Can you work these out from the drawing? Everything is in mm from the part's minimum corner. Coordinates: 2 decimals unless noted, no trailing zeros. Order: outer loops, then holes, each group sorted by start corner. A loop starts at its lowest first (then second) coordinate and runs counter-clockwise, first axis right, second up. Notation, with made-up numbers: (29.5, 39) -> (54.5, 39) arc R30 cw to (54.5, 71) -> close; hole circle Ø7 at (71, 56.25). An arc over 180 degrees is marked (long way). Return JSON: item names as keys, results as strings. Group by question number.
1) If I drill on probe 1 along X at (y, z) = (5.75, 35.5) (1 decimal); probe 2 along X at (y, z) = (1.5, 33.5) (1 decimal); probe 3 along X at (y, z) = (10.5, 38) (1 decimal), over which ranges is the centre line in solid material (lowest first)? Write a range as from..to.
2) For pin 1 (3 mm diameter, centred on x = 49.5, y = 11.5, fed in from +Z) (1 decimal); pin 2 (5 mm diameter, centred on y = 2.5, z = 52.5, fed in from +X); pin 3 (1.5 mm diameter, centred on y = 6, z = 30.5, fed in from -X), each with a flat end and sliding along its axis, tell me the tip position at first contact or that it passes through.
3) If we section it at B-B, the plane y = 12.25: Please give me the cut outline in (x, z).
4) Thinking about a two-plate mould opening in X: for the marked faces 1, 2 and 3, which applies, +X half, -X half, draft (parallel to the pull), parting line (faces both ways), or undercut?
5) If we section it at A-A, the plane y = 1.25: Please give me the cut outline in (x, z) (1 decimal), then the cut area to 3 significant figures.
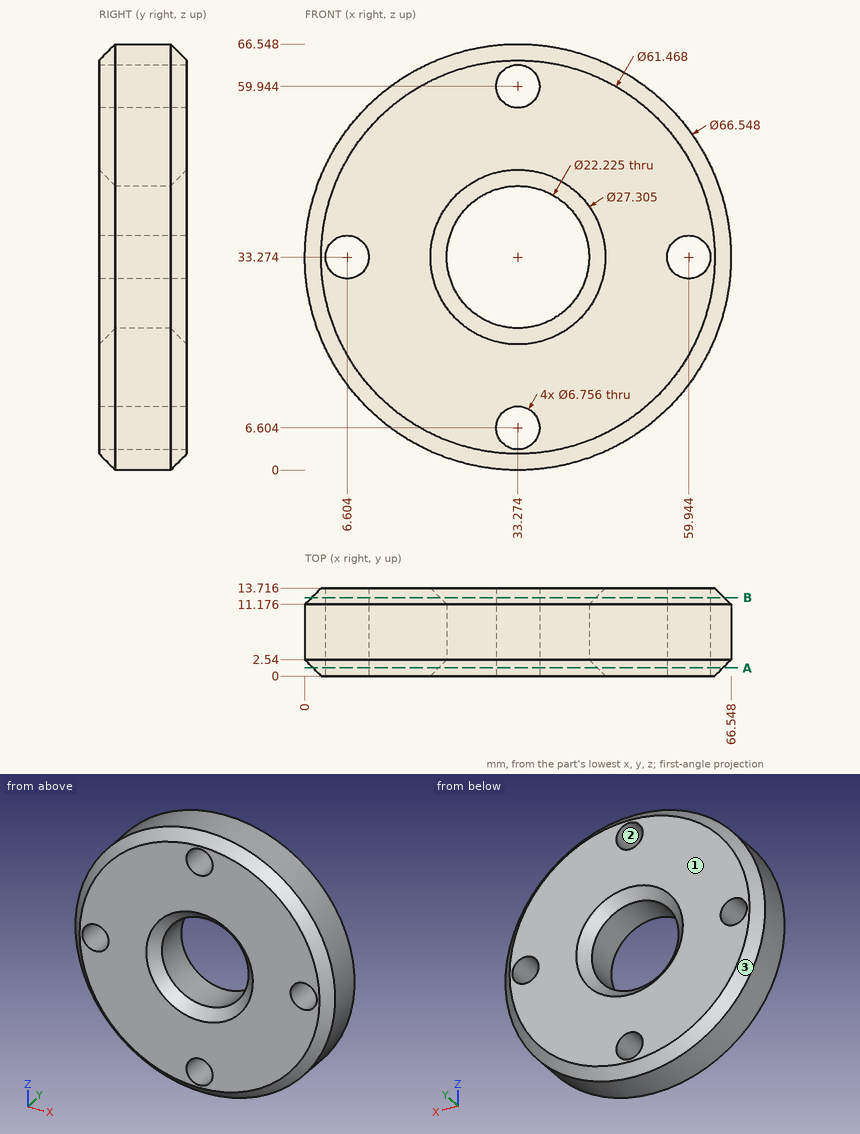
Result sheet:
{
 "1": {"probe 1": "x = 0.1..4.1, 9.1..22.4, 44.2..57.4, 62.5..66.5", "probe 2": "x = 1..3.2, 10..21.1, 45.4..56.6, 63.3..65.5", "probe 3": "x = 0.3..23.2, 43.3..66.2"},
 "2": {"pin 1": "stops at z = 63.1", "pin 2": "stops at x = 62.04", "pin 3": "stops at x = 0.06"},
 "3": {"outline": "circle Ø64.4 at (33.27, 33.27); hole circle Ø6.76 at (6.6, 33.27); hole circle Ø24.37 at (33.27, 33.27); hole circle Ø6.76 at (33.27, 6.6); hole circle Ø6.76 at (33.27, 59.94); hole circle Ø6.76 at (59.94, 33.27)"},
 "4": {"face 1": "draft", "face 2": "undercut", "face 3": "parting line"},
 "5": {"outline": "circle Ø64 at (33.3, 33.3); hole circle Ø6.8 at (6.6, 33.3); hole circle Ø24.8 at (33.3, 33.3); hole circle Ø6.8 at (33.3, 6.6); hole circle Ø6.8 at (33.3, 59.9); hole circle Ø6.8 at (59.9, 33.3)", "area": "2,590 mm2"}
}
